```python
from build123d import *

# Parameters (mm, degrees)
F3_W     = 101.6
F3_H     = 101.6
F4_DEPTH = 50.8
F0_R     = 25.4
F5_DEPTH = 101.601
F1_R     = 12.7
F2_DEPTH = 101.6


with BuildPart() as f4:
    # F3 (on Front) → F4 (new body, symmetric)
    with BuildSketch(Plane.XZ):
        Rectangle(F3_W, F3_H)
    extrude(amount=F4_DEPTH, both=True)

    # F0 (on face) → F5 (cut, through all)
    with BuildSketch(Plane(origin=(-50.8, 0, 0), x_dir=(0, -1, 0), z_dir=(-1, 0, 0))):
        Circle(F0_R)
    extrude(amount=-F5_DEPTH, mode=Mode.SUBTRACT)

    # F1 (on face) → F2 (join)
    with BuildSketch(Plane.XY.offset(50.8)):
        Circle(F1_R)
    extrude(amount=-F2_DEPTH)


solid = f4.part
```
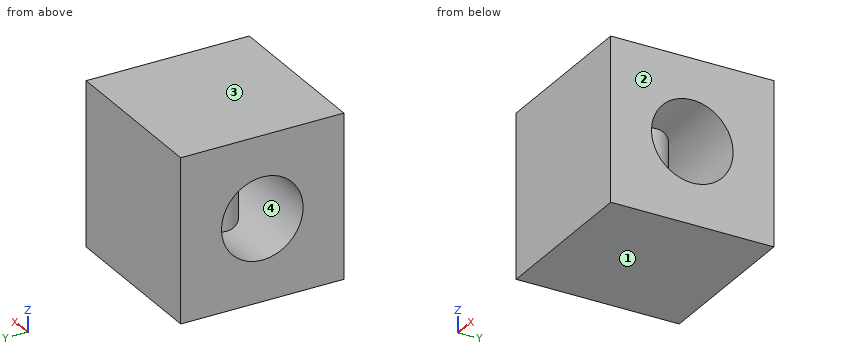
Part model, mm, in its own coordinate system. Face numbers are marked on the shaded views. Round coordinates to 2 decimals unless told otherwise and drop trailing zeros. Loops run counter-clockwise (first coordinate to the right, second up) from the corner with the lowest first, then second, coordinate; pieces in that order, holes last. Notation, with made-up numbers: (85, 44.5) -> (98, 44.5) arc R15 cw to (98, 51.5) -> close; hole circle Ø4 at (-25.75, -3). An arc over 180 degrees is marked (long way). Use CSV: the item, a comma, the result in double quotes. Start each with the question number.
1) Wall check: L1, parallel to Z at x = 14, y = 0; L2, parallel to Y at x = -28.5, z = 15.5; L3, parallel to Z at x = 36, y = 21. Give the ranges that are in metal, low to high. Write a range as [from, to].
2) Cut at A-A, the plane z = 0. Write the cut outline in (x, y).
3) Cut at D-D, the plane x = -9. Write the cut outline in (y, z), plus the area to 3 significant figures.
4) Pull direction Z, two halves, no side cores. Call the marked faces 1, 2, 3 and 4: +Z half, -Z half, draft (parallel to the pull), parting line (faces both ways), or undercut.
5) Cut at C-C, the plane x = -32. Write the cut outline in (y, z).
6) Cut at B-B, the plane y = 0. Write the cut outline in (x, z).
7) Drop a flat-ended pin along its axis: P1, Ø1, axis at y = -5, z = -2.5, coming from the -X side. Give the stop position or say it passes through.
Determined:
1,L1,"z = [-50.8, -25.4], [25.4, 50.8]"
1,L2,"y = [-50.8, -20.12], [20.12, 50.8]"
1,L3,"z = [-50.8, -14.29], [14.29, 50.8]"
2,outline,"(-50.8, -50.8) -> (50.8, -50.8) -> (50.8, -25.4) -> (-50.8, -25.4) -> close; (-50.8, 25.4) -> (50.8, 25.4) -> (50.8, 50.8) -> (-50.8, 50.8) -> close; circle Ø25.4 at (0, 0)"
3,outline,"(-50.8, -50.8) -> (50.8, -50.8) -> (50.8, 50.8) -> (-50.8, 50.8) -> close; hole (-8.96, -23.77) -> (-8.96, 23.77) arc R25.4 ccw to start; hole (8.96, -23.77) arc R25.4 ccw to (8.96, 23.77) -> close"
3,area,"9,190 mm2"
4,face 1,"-Z half"
4,face 2,"draft"
4,face 3,"+Z half"
4,face 4,"undercut"
5,outline,"(-50.8, -50.8) -> (50.8, -50.8) -> (50.8, 50.8) -> (-50.8, 50.8) -> close; hole circle Ø50.8 at (0, 0)"
6,outline,"(-50.8, -50.8) -> (50.8, -50.8) -> (50.8, -25.4) -> (12.7, -25.4) -> (12.7, 25.4) -> (50.8, 25.4) -> (50.8, 50.8) -> (-50.8, 50.8) -> (-50.8, 25.4) -> (-12.7, 25.4) -> (-12.7, -25.4) -> (-50.8, -25.4) -> close"
7,P1,"stops at x = -11.88"
